Work out the finished part from the listing and answer in its coordinate system (mm). Face numbers are marked on the shaded views. A direction names the side the tool comes from. Round coordinates to 2 decimals unless told otherwise and drop trailing zeros. Loops run counter-clockwise (first coordinate to the right, second up) from the corner with the lowest first, then second, coordinate; pieces in that order, holes last. Notation, with made-up numbers: (40.5, 17) - (61.5, 17) arc R13 cw to (61.5, 27) - close; hole circle Ø4 at (85.25, 48.5). An arc over 180 degrees is marked (long way). Answer as CSV lines item,"result". Start each with the question number.
Q1. The mould has two halves that part along Y. Classify the marked faces 3, 4 and 5: +Y half, -Y half, draft (parallel to the pull), parting line (faces both ways), or undercut.
Q2. Straight lines are drawn through the part: L1, parallel to Y at x = 1.2, z = 0; L2, parallel to X at y = -10.5, z = -4.5; L3, parallel to Y at x = 3.75, z = 0. For each, find the intervals that lie inside material, in ascending order. Write a range as [from, to].
Q3. Section C-C on y = 10 is taken. Write down the section's boundary in (x, z).
Q4. Section D-D on z = -4 is taken. Write down the section's boundary in (x, y), then the cut area to 3 significant figures.
Q5. Each of these flat-tipped pins is pushed along its axis until it touches: pin 1 Ø1.5 at (y, z) = (3, -0.5) entering from +X; pin 2 Ø1.5 at (y, z) = (-5, -2.5) entering from -X; pin 3 Ø2 at (x, z) = (4.5, -1.5) entering from -Y; pin 4 Ø2 at (x, z) = (9.5, 2) entering from +Y. Where does it stop, or does it pass through?
Q6. For the marked faces 1 and 2, determine the directions among +Z, -Z, +X, -X, +Y, -Y from which every point of the face is accessible in a straight line to the end or side of a thin tool.
Q7. Section A-A on y = -10 is taken. Write down the section's boundary in (x, z), then the cut area to 3 significant figures.
Q8. Section B-B on z = 0 is taken. Write down the section's boundary in (x, y).
```python
from build123d import *

# Parameters (mm, degrees)
SKETCH1_W           = 10
SKETCH1_H           = 30
BOSS_EXTRUDE1_DEPTH = 2
SKETCH2_R           = 3.5
CUT_EXTRUDE1_DEPTH  = 2
SKETCH3_R           = 3
BOSS_EXTRUDE2_DEPTH = 10


with BuildPart() as part:
    # Sketch1 → Boss-Extrude1 (new body)
    with BuildSketch(Plane(origin=(0, 0, 0), x_dir=(0, 0, -1), z_dir=(1, 0, 0))):
        Rectangle(SKETCH1_W, SKETCH1_H)
    extrude(amount=BOSS_EXTRUDE1_DEPTH)

    # Sketch2 → Cut-Extrude1 (cut)
    with BuildSketch(Plane(origin=(2, 0, 0), x_dir=(0, 0, -1), z_dir=(1, 0, 0))):
        with Locations((0, -10)):
            Circle(SKETCH2_R)
    extrude(amount=-CUT_EXTRUDE1_DEPTH, mode=Mode.SUBTRACT)

    # Sketch3 → Boss-Extrude2 (add)
    with BuildSketch(Plane(origin=(2, 0, 0), x_dir=(0, 0, -1), z_dir=(1, 0, 0))):
        with Locations((0, 10)):
            Circle(SKETCH3_R)
    extrude(amount=BOSS_EXTRUDE2_DEPTH)


solid = part.part
```
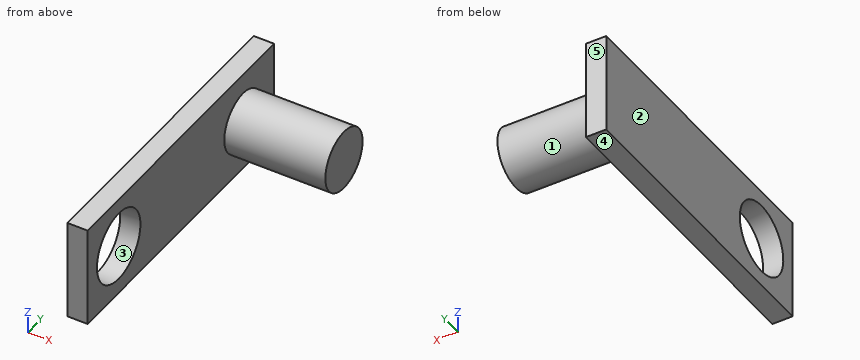
Findings:
1,face 3,"undercut"
1,face 4,"draft"
1,face 5,"+Y half"
2,L1,"y = [-15, -13.5], [-6.5, 15]"
2,L2,"x = [0, 2]"
2,L3,"y = [7, 13]"
3,outline,"(0, -5) - (2, -5) - (2, -3) - (12, -3) - (12, 3) - (2, 3) - (2, 5) - (0, 5) - close"
4,outline,"(0, -15) - (2, -15) - (2, 15) - (0, 15) - close"
4,area,"60.0 mm^2"
5,pin 1,"stops at x = 2"
5,pin 2,"stops at x = 0"
5,pin 3,"stops at y = 7.04"
5,pin 4,"stops at y = 12.83"
6,face 1,"+X"
6,face 2,"+Z, -Z, -X, +Y, -Y"
7,outline,"(0, -5) - (2, -5) - (2, -3.5) - (0, -3.5) - close; (0, 3.5) - (2, 3.5) - (2, 5) - (0, 5) - close"
7,area,"6.00 mm^2"
8,outline,"(0, -15) - (2, -15) - (2, -13.5) - (0, -13.5) - close; (0, -6.5) - (2, -6.5) - (2, 7) - (12, 7) - (12, 13) - (2, 13) - (2, 15) - (0, 15) - close"
